Autodesk Inventor part; units mm, degrees
ref_plane "YZ Plane" through (0, 0, 0) normal (1, 0, 0) x (0, 1, 0)
ref_plane "XZ Plane" through (0, 0, 0) normal (0, 1, 0) x (-1, 0, 0)
ref_plane "XY Plane" through (0, 0, 0) normal (0, 0, 1) x (1, 0, 0)
sketch "Sketch1" plane through (0, 0, 0) normal (0, 0, 1) x (1, 0, 0)
  circle A0 centre (91.8298, -26) radius 2.15
  circle A1 centre (91.8298, 26) radius 2.15
  line L0 (1.8298, 37) -> (-37.1702, 37)
  line L1 (-37.1702, 37) -> (-37.1702, -37)
  line L2 (-37.1702, -37) -> (1.8298, -37)
  circle A2 centre (-4.1702, -32) radius 2.15
  circle A3 centre (-31.1702, -32) radius 2.15
  circle A4 centre (-31.1702, 32) radius 2.15
  circle A5 centre (-4.1702, 32) radius 2.15
  line L3 (-9.9952, 18) -> (35.6548, 18)
  line L4 (38.8298, 14.825) -> (38.8298, -14.825)
  line L5 (35.6548, -18) -> (-9.9952, -18)
  line L6 (-13.1702, -14.825) -> (-13.1702, 14.825)
  arc A6 (-9.9952, 18) -> (-13.1702, 14.825) centre (-9.9952, 14.825) ccw
  arc A7 (-13.1702, -14.825) -> (-9.9952, -18) centre (-9.9952, -14.825) ccw
  arc A8 (38.8298, 14.825) -> (35.6548, 18) centre (35.6548, 14.825) ccw
  arc A9 (35.6548, -18) -> (38.8298, -14.825) centre (35.6548, -14.825) ccw
  line L7 (85.8298, 28.175) -> (85.8298, 30)
  line L8 (85.8298, 30) -> (97.8298, 30)
  line L9 (97.8298, 30) -> (97.8298, -30)
  line L10 (85.8298, -28.175) -> (85.8298, -30)
  line L11 (85.8298, -30) -> (97.8298, -30)
  arc A10 (82.6548, 25) -> (85.8298, 28.175) centre (82.6548, 28.175) ccw
  arc A11 (85.8298, -28.175) -> (82.6548, -25) centre (82.6548, -28.175) ccw
  line L12 (1.8298, 37) -> (1.8298, 28.175)
  line L13 (5.0048, 25) -> (82.6548, 25)
  line L14 (1.8298, -37) -> (1.8298, -28.175)
  line L15 (5.0048, -25) -> (82.6548, -25)
  arc A12 (1.8298, 28.175) -> (5.0048, 25) centre (5.0048, 28.175) ccw
  arc A13 (5.0048, -25) -> (1.8298, -28.175) centre (5.0048, -28.175) ccw
  point P0 (0, 0)
  point P1 (85.8298, 26.8)
  dimension "d2" = 4.3
  dimension "d3" = 4.3
  dimension "d20" = 6
  dimension "d21" = 6
  dimension "d23" = 4.3
  dimension "d24" = 4.3
  dimension "d25" = 4.3
  dimension "d26" = 4.3
  dimension "d41" = 3.175
  dimension "d53" = 6
  dimension "d54" = 6
  dimension "d55" = 6
  dimension "d57" = 3.175
  dimension "d63" = 84
  dimension "d64" = 3.175
  dimension "d65" = 3.175
  dimension "d68" = 84
  dimension "d69" = 36
  dimension "d70" = 52
  dimension "d75" = 6
  dimension "d76" = 6
  dimension "d78" = 12
  dimension "d79" = 39
  dimension "d80" = 24
  dimension "d81" = 7
  dimension "d82" = 7
  dimension "d83" = 74
  dimension "d84" = 12
  dimension "d85" = 5
  dimension "d86" = 5
  dimension "d87" = 5
  dimension "d88" = 5
  dimension "d89" = 37
  dimension "d90" = 52
  dimension "d92" = 26
  dimension "d93" = 25
  dimension "d94" = 25
  dimension "d95" = 4
  dimension "d96" = 4
extrude "Extrusion5" add sketch "Sketch1" along normal blind 2
equation "\"d3\" = d2"
equation "\"d24\" = d23"
equation "\"d25\" = d23"
equation "\"d26\" = d23"
equation "\"d55\" = d53"
equation "\"d68\" = d63"
equation "\"d75\" = d19"
equation "\"d76\" = d19"
properties part number "bottom support extension"
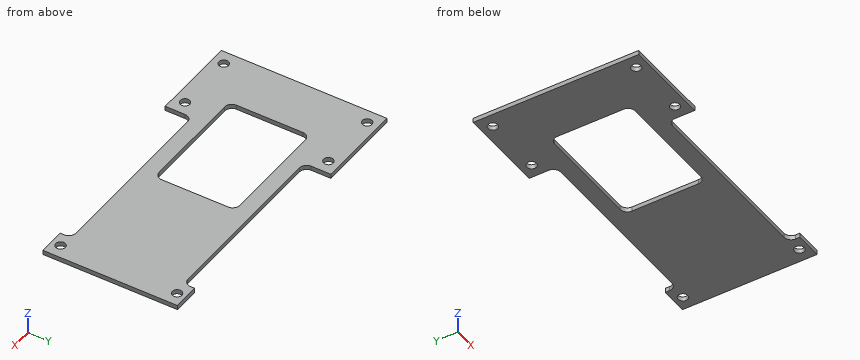
The listing builds one solid part. Answer for the finished solid, in the listing's coordinates (mm). Round coordinates to 2 decimals unless told otherwise and drop trailing zeros. Loops run counter-clockwise (first coordinate to the right, second up) from the corner with the lowest first, then second, coordinate; pieces in that order, holes last. Notation, with made-up numbers: M 27.5,-16.75 L 83.5,-16.75 A22 cw 83.5,10.25 Z; hole C 45,43.25 d6. An arc over 180 degrees is marked long. Return JSON: item names as keys, results as strings.
Q1. Find the intervals of material crossed by line 1 along Y through (x, z) = (30.5, 0.55); line 2 along X through (y, z) = (0, 1.35); line 3 along X through (y, z) = (27.5, 1.7), in increasing order. Write a range as from..to.
Results list:
{"line 1": "y = -25..-18, 18..25", "line 2": "x = -37.17..-13.17, 38.83..97.83", "line 3": "x = -37.17..1.9, 85.76..90.29, 93.37..97.83"}
Q2. Find section C-C, the plane z = 1. State how many separate pieces and enclosed holes the cut face has, plus the area to 3 significant figures.
Results list:
{"separate pieces": "1", "enclosed holes": "7", "area": "5,860 mm2"}
Q3. Each of these flat-tipped pins is pushed along its axis until it touches: pin 1 Ø1 at (y, z) = (-34, 1) entering from +X; pin 2 Ø1 at (x, z) = (94, 1.5) entering from +Y; pin 3 Ø5 at (x, y) = (25.5, 23) entering from -Z. Where does it stop, or does it pass through?
Results list:
{"pin 1": "stops at x = 1.83", "pin 2": "stops at y = 30", "pin 3": "stops at z = 0"}
Q4. Find section D-D, the plane y = 9.5. Determine the outline of the cut face in (x, z).
Results list:
{"outline": "M -37.17,0 L -13.17,0 L -13.17,2 L -37.17,2 Z; M 38.83,0 L 97.83,0 L 97.83,2 L 38.83,2 Z"}
Q5. Find section A-A, the plane x = 21. Determine the outline of the cut face in (y, z), plus the area to 3 significant figures.
Results list:
{"outline": "M -25,0 L -18,0 L -18,2 L -25,2 Z; M 18,0 L 25,0 L 25,2 L 18,2 Z", "area": "28.0 mm2"}
Q6. Find section B-B, the plane y = -32. Determine the outline of the cut face in (x, z).
Results list:
{"outline": "M -37.17,0 L -33.32,0 L -33.32,2 L -37.17,2 Z; M -29.02,0 L -6.32,0 L -6.32,2 L -29.02,2 Z; M -2.02,0 L 1.83,0 L 1.83,2 L -2.02,2 Z"}
